from build123d import *

# Parameters (mm, degrees)
SKETCH_R        = 55
PAD_DEPTH       = 4
SKETCH003_R     = 1.3
POCKET001_DEPTH = 5
SKETCH004_R     = 1.3
POCKET_DEPTH    = 5
SKETCH005_R     = 1.8
POCKET002_DEPTH = 5


with BuildPart() as part:
    # Sketch → Pad (new body)
    with BuildSketch(Plane.XY):
        Circle(SKETCH_R)
    extrude(amount=PAD_DEPTH)

    # Sketch003 → Pocket001 (cut)
    with BuildSketch(Plane.XY.offset(4)):
        with Locations((-44, -20)):
            Circle(SKETCH003_R)
        with Locations((44, 20)):
            Circle(SKETCH003_R)
    extrude(amount=-POCKET001_DEPTH, mode=Mode.SUBTRACT)

    # Sketch004 (on Face3 of Pocket001) → Pocket (cut)
    with BuildSketch(Plane.XY.offset(4)):
        with Locations((3, -50)):
            Circle(SKETCH004_R)
        with Locations((-3, -50)):
            Circle(SKETCH004_R)
        with Locations((-3, 50)):
            Circle(SKETCH004_R)
        with Locations((3, 50)):
            Circle(SKETCH004_R)
    extrude(amount=-POCKET_DEPTH, mode=Mode.SUBTRACT)

    # Sketch005 (on Face2 of Pocket) → Pocket002 (cut)
    with BuildSketch(Plane(origin=(0, 0, 0), x_dir=(1, 0, 0), z_dir=(0, 0, -1))):
        with Locations((17.262171, 32.243663)):
            Circle(SKETCH005_R)
        with Locations((17.262171, -7.756337)):
            Circle(SKETCH005_R)
        with Locations((5.258312, 39.084725)):
            Circle(SKETCH005_R)
        with Locations((-43.741688, -18.915275)):
            Circle(SKETCH005_R)
        with Locations((5.258312, -18.915275)):
            Circle(SKETCH005_R)
    extrude(amount=-POCKET002_DEPTH, mode=Mode.SUBTRACT)


solid = part.part
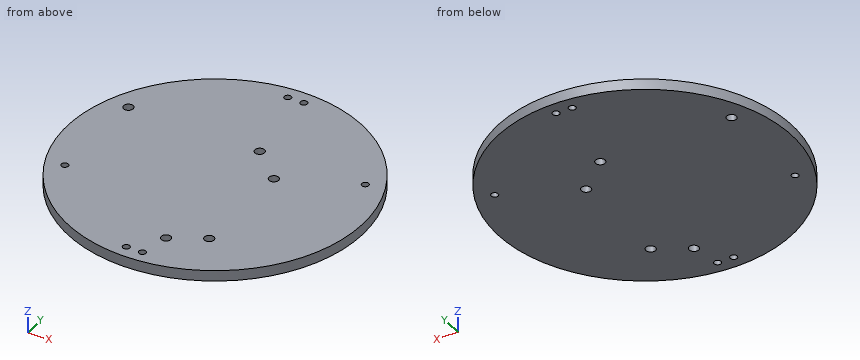
The model under review builds one solid part; all positions refer to its coordinate system, in mm. Give positions to 0.01 mm unless a question says otherwise; leave off trailing zeros. Order: outer loops, then holes, each group sorted by start corner. A loop starts at its lowest first (then second) coordinate and runs counter-clockwise, first axis right, second up. Notation, with made-up numbers: (-21.75, -18) -> (35.25, -18) arc R19 cw to (35.25, -13) -> close; hole circle Ø6 at (28, -23.5). An arc over 180 degrees is marked (long way). Write item = value, one per line. Start each with the question number.
(1) For pin 1 Ø4.5 at (x, y) = (5.26, 18.92) entering from +Z; pin 2 Ø3 at (x, y) = (17.26, 7.76) entering from +Z, all flat-tipped, find the tip position at first contact; note any pin that passes through.
(2) Take a section at B-B (y = 50). Write out the cut boundary in (x, z), plus the area to 3 significant figures.
(3) Take a section at D-D (x = -3). Write out the cut boundary in (y, z), plus the area to 3 significant figures.
(4) For L1, parallel to Y at x = -44, z = 3.45; L2, parallel to Y at x = -3, z = 2.4; L3, parallel to Y at x = -0.5, z = 1.1, list the stretches that pass through material, from the lowest coordinate up. Write a range as from..to.
(5) Take a section at A-A (x = 44). Write out the cut boundary in (y, z), plus the area to 3 significant figures.
(6) Take a section at C-C (z = 1.35). State how many separate pieces and enclosed holes the cut face has, plus the area to 3 significant figures.
Returned:
q1.pin_1 = 4
q1.pin_2 = through
q2.outline = (-22.91, 0) -> (-4.3, 0) -> (-4.3, 4) -> (-22.91, 4) -> close; (-1.7, 0) -> (1.7, 0) -> (1.7, 4) -> (-1.7, 4) -> close; (4.3, 0) -> (22.91, 0) -> (22.91, 4) -> (4.3, 4) -> close
q2.area = 163 mm²
q3.outline = (-54.92, 0) -> (-51.3, 0) -> (-51.3, 4) -> (-54.92, 4) -> close; (-48.7, 0) -> (48.7, 0) -> (48.7, 4) -> (-48.7, 4) -> close; (51.3, 0) -> (54.92, 0) -> (54.92, 4) -> (51.3, 4) -> close
q3.area = 419 mm²
q4.L1 = -33..-21.3, -18.7..17.13, 20.7..33
q4.L2 = -54.92..-51.3, -48.7..48.7, 51.3..54.92
q4.L3 = -55..55
q5.outline = (-33, 0) -> (18.7, 0) -> (18.7, 4) -> (-33, 4) -> close; (21.3, 0) -> (33, 0) -> (33, 4) -> (21.3, 4) -> close
q5.area = 254 mm²
q6.separate_pieces = 1
q6.enclosed_holes = 11
q6.area = 9,420 mm²
